The model under review builds one solid part; all positions refer to its coordinate system, in mm. A direction names the side the tool comes from. Round coordinates to 2 decimals unless told otherwise and drop trailing zeros. Loops run counter-clockwise (first coordinate to the right, second up) from the corner with the lowest first, then second, coordinate; pieces in that order, holes last. Notation, with made-up numbers: (55.5, -21.5) -> (74.5, -21.5) arc R12 cw to (74.5, 0.5) -> close; hole circle Ø2 at (48.25, 58). An arc over 180 degrees is marked (long way). Use a Markdown table: item, result. Add a question column.
1) Mouldability with a two-part tool opening along Z and no side actions: class faces 3 (the flat face through (-74, 2032, 34)), 4 (the flat face through (-1, 1002, 76.2)), 5 (the flat face through (-1, 1002, 73.66)) as released by +Z, released by -Z, zero draft, split by the parting line, or undercut.
2) Consider section B-B on z = -48.5. Give the boundary of the cut face in (x, y).
3) For faces 1 (the flat face through (-1, 1002, -73.66)), 2 (the flat face through (76.2, 1002, 1)), list the 3-axis set-ups (+Z, -Z, +X, -X, +Y, -Y) from which the entire face can be reached by the end or side of a thin tool; tool diameter is ignored.
4) Consider section A-A on x = 55. Give the boundary of the cut face in (y, z).
5) Consider section C-C on y = 1211. Give the boundary of the cut face in (x, z).
6) Wall thickness on probe 1 along X at (y, z) = (1620.5, -36): over which ranges is the line inside the solid? List them lowest first.
from build123d import *

# Parameters (mm, degrees)
SKETCH1_W           = 152.4
SKETCH1_H           = 152.4
SKETCH1_W_2         = 147.32
SKETCH1_H_2         = 147.32
BOSS_EXTRUDE1_DEPTH = 6604
SKETCH2_W           = 152.4
SKETCH2_H           = 4572
CUT_EXTRUDE1_DEPTH  = 6607.197711241


with BuildPart() as part:
    # Sketch1 → Boss-Extrude1 (new body)
    with BuildSketch(Plane(origin=(0, 0, 0), x_dir=(1, 0, 0), z_dir=(0, 1, 0))):
        Rectangle(SKETCH1_W, SKETCH1_H)
        Rectangle(SKETCH1_W_2, SKETCH1_H_2, mode=Mode.SUBTRACT)
    extrude(amount=BOSS_EXTRUDE1_DEPTH)

    # Sketch2 → Cut-Extrude1 (cut, through all)
    with BuildSketch(Plane.XY.offset(76.2)):
        with Locations((0, 4318)):
            Rectangle(SKETCH2_W, SKETCH2_H)
    extrude(amount=-CUT_EXTRUDE1_DEPTH, mode=Mode.SUBTRACT)


solid = part.part
Result set:
| question | item | result |
|---|---|---|
| 1 | face 3 | zero draft |
| 1 | face 4 | released by +Z |
| 1 | face 5 | undercut |
| 2 | outline | (-76.2, 0) -> (-73.66, 0) -> (-73.66, 2032) -> (-76.2, 2032) -> close; (73.66, 0) -> (76.2, 0) -> (76.2, 2032) -> (73.66, 2032) -> close |
| 3 | face 1 | +Y, -Y |
| 3 | face 2 | +Z, -Z, +X, +Y, -Y |
| 4 | outline | (0, -76.2) -> (2032, -76.2) -> (2032, -73.66) -> (0, -73.66) -> close; (0, 73.66) -> (2032, 73.66) -> (2032, 76.2) -> (0, 76.2) -> close |
| 5 | outline | (-76.2, -76.2) -> (76.2, -76.2) -> (76.2, 76.2) -> (-76.2, 76.2) -> close; hole (-73.66, -73.66) -> (73.66, -73.66) -> (73.66, 73.66) -> (-73.66, 73.66) -> close |
| 6 | probe 1 | -76.2 to -73.66, 73.66 to 76.2 |
